Input: part model. Units: mm. Frame: model coordinates. Coordinates: 2 decimals unless noted, no trailing zeros. Loops run counter-clockwise (first coordinate to the right, second up) from the corner with the lowest first, then second, coordinate; pieces in that order, holes last.
```python
from build123d import *

# Parameters (mm, degrees)
F2_DEPTH = 1
F0_W     = 55
F0_H     = 55
F3_DEPTH = 28


with BuildPart() as f2:
    # F1 (on face) → F2 (new body)
    with BuildSketch(Plane.XY):
        Polygon((1, -1), (54, -1), (54, -55), (55.060755, -55), (55.060755, 0), (0, 0), (0, -55), (1, -55), align=None)
    extrude(amount=F2_DEPTH)

    # F0 (on Top) → F3 (join)
    with BuildSketch(Plane.XY):
        with Locations((27.5, -27.5)):
            Rectangle(F0_W, F0_H)
    extrude(amount=-F3_DEPTH)


solid = f2.part
```
Item 1: Section query B-B (x = 17). Output: boundary loops of the cut face in (y, z).
Result:
outline: (-55, -28) - (0, -28) - (0, 1) - (-1, 1) - (-1, 0) - (-55, 0) - close
Item 2: Contact query for flat-ended pins moving along their axis: P1, Ø12, axis at x = 10, y = -16.5, coming from the +Z side; P2, Ø14, axis at y = -38, z = -11.5, coming from the +X side; P3, Ø0.5, axis at x = 32.5, z = 0.5, coming from the -Y side. Output: stop coordinate, or through.
Result:
P1: stops at z = 0
P2: stops at x = 55
P3: stops at y = -1
Item 3: Mould query, pull axis X, two halves, no side actions, for faces 1 (the face through (0, -28, -13)), 2 (the face through (27, -28, 0)), 3 (the face through (55, -28, -14)). Classes: +X half, -X half, draft (parallel to the pull), parting line (faces both ways), or undercut.
Result:
face 1: -X half
face 2: undercut
face 3: +X half
Item 4: Section query A-A (y = -32). Output: boundary loops of the cut face in (x, z).
Result:
outline: (0, -28) - (55, -28) - (55, 0) - (55.06, 0) - (55.06, 1) - (54, 1) - (54, 0) - (1, 0) - (1, 1) - (0, 1) - close
Item 5: Line query: L1, parallel to X at y = -26, z = -11.75; L2, parallel to Z at x = 46.5, y = -37. Output: solid intervals per line, ascending.
Result:
L1: x = 0 to 55
L2: z = -28 to 0
